Check sheet for the drawn part. Datum: minimum x, y, z corner. Units: mm. Round coordinates to 2 decimals unless told otherwise and drop trailing zeros. Write each loop counter-clockwise with the first axis right and the second up, starting at its lowest first coordinate (ties: lowest second). Pieces come first, ordered by that corner, then holes.
Item 1: Cross-section at A-A on z = 21. Enter the section's corners in (x, y).
Item 2: Go/stop test with a flat-tipped pin: pin 1 Ø4 at (x, z) = (30.5, 67.5) entering from +Y. Record where the tip stops, or that it passes through.
Item 3: Cross-section at B-B on x = 44.5. Enter the section's corners in (y, z).
Item 4: Cross-section at D-D on x = 13. Enter the section's corners in (y, z).
Item 5: Material ranges on line 1 (Z direction, x = 45, y = 4.75); line 2 (X direction, y = 3.4, z = 75.5); line 3 (Y direction, x = 33, z = 65.5), recorded low to high.
Item 6: Cross-section at C-C on y = 4. Enter the section's corners in (x, z), plus the area to 3 significant figures.
Item 7: Release check for a two-part mould opening along X. For the marked faces 1 and 2 record: +X half, -X half, draft (parallel to the pull), parting line (faces both ways), or undercut.
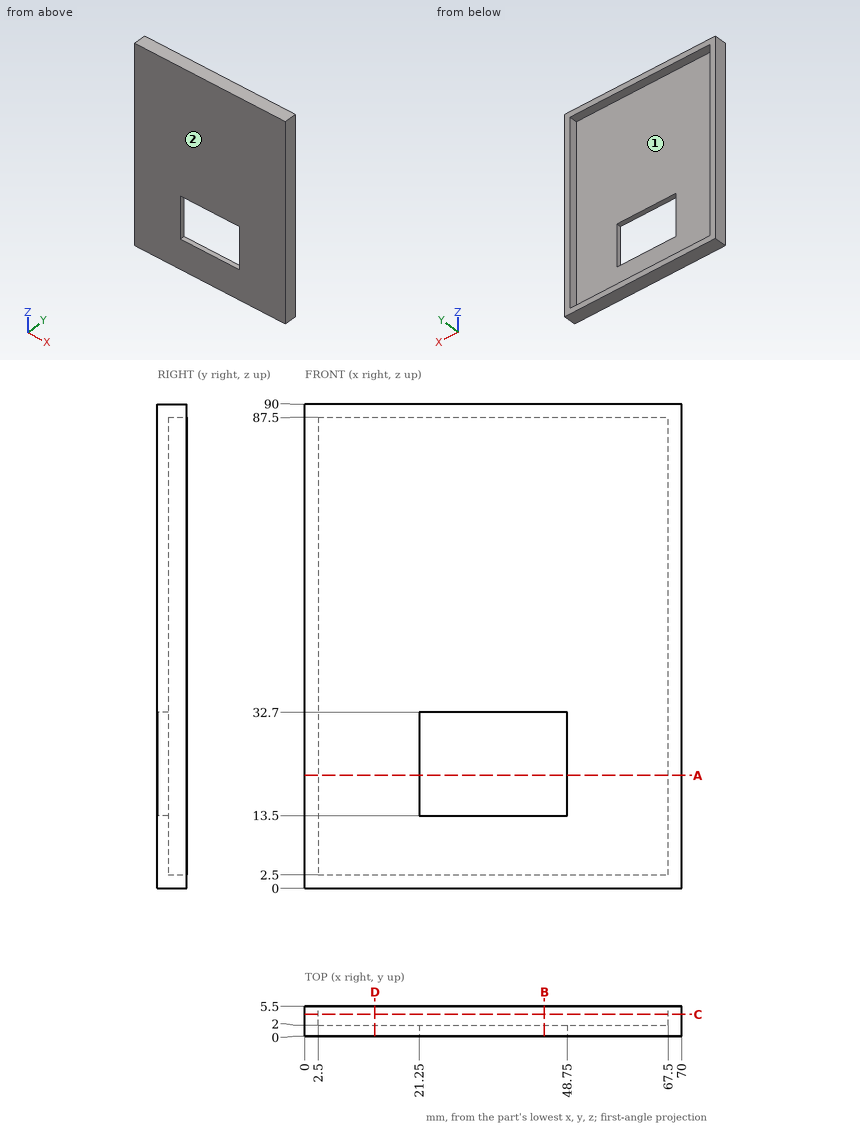
Response values:
1. outline: (0, 0) - (21.25, 0) - (21.25, 2) - (2.5, 2) - (2.5, 5.5) - (0, 5.5) - close; (48.75, 0) - (70, 0) - (70, 5.5) - (67.5, 5.5) - (67.5, 2) - (48.75, 2) - close
2. pin 1: stops at y = 2
3. outline: (0, 0) - (5.5, 0) - (5.5, 2.5) - (2, 2.5) - (2, 13.5) - (0, 13.5) - close; (0, 32.7) - (2, 32.7) - (2, 87.5) - (5.5, 87.5) - (5.5, 90) - (0, 90) - close
4. outline: (0, 0) - (5.5, 0) - (5.5, 2.5) - (2, 2.5) - (2, 87.5) - (5.5, 87.5) - (5.5, 90) - (0, 90) - close
5. line 1: z = 0 to 2.5, 87.5 to 90
5. line 2: x = 0 to 2.5, 67.5 to 70
5. line 3: y = 0 to 2
6. outline: (0, 0) - (70, 0) - (70, 90) - (0, 90) - close; hole (2.5, 2.5) - (67.5, 2.5) - (67.5, 87.5) - (2.5, 87.5) - close
6. area: 775 mm2
7. face 1: undercut
7. face 2: draft
